The listing builds one solid part. Answer for the finished solid, in the listing's coordinates (mm). Face numbers are marked on the shaded views. A direction names the side the tool comes from. Give positions to 0.01 mm unless a question says otherwise; leave off trailing zeros. Order: outer loops, then holes, each group sorted by start corner. A loop starts at its lowest first (then second) coordinate and runs counter-clockwise, first axis right, second up. Notation, with made-up numbers: (-19, 64) - (-9, 64) arc R12 ccw to (-9, 80) - close; hole circle Ø11 at (13.25, -21). An arc over 180 degrees is marked (long way). Use CSV: the item, a comma, the result in double quotes.
```python
from build123d import *

# Parameters (mm, degrees)
FILLET1_R                     = 1
CHAMFER1_SIZE                 = 1.016
CHAMFER2_SIZE                 = 0.5
F_10_32_TAPPED_HOLE1_D        = 4.0386
F_10_32_TAPPED_HOLE1_DEPTH    = 13.6144
F_10_32_TAPPED_HOLE1_TIP      = 1.213317848
CUT_EXTRUDE1_START            = -6.79958
CUT_EXTRUDE1_DEPTH            = 122.301029095
SKETCH5_R                     = 4.318
BOSS_EXTRUDE1_DEPTH           = 2.2606
BOSS_EXTRUDE1_DRAFT           = 45
BOSS_EXTRUDE1_PROFILE_2_DEPTH = 2.2606
BOSS_EXTRUDE1_PROFILE_2_DRAFT = 45


with BuildPart() as part:
    # Sketch1 → Revolve1 (revolve)
    with BuildSketch(Plane(origin=(0, 0, 0), x_dir=(0, 0, -1), z_dir=(1, 0, 0)), mode=Mode.PRIVATE) as revolve1_sk:
        Polygon((-31.623, 0), (-31.623, 3.9751), (0, 3.9751), (0, 9.525), (3.9878, 9.525), (3.9878, 31.877), (12.2174, 31.877), (12.2174, 32.2072), (105.3592, 32.2072), (105.3592, 31.877), (113.5888, 31.877), (113.5888, 15.0368), (118.5888, 15.0368), (118.5888, 0), align=None)
    revolve(revolve1_sk.sketch.rotate(Axis((0, 0, 111.866494726), (0, 0, -1)), 90), axis=Axis((0, 0, 111.866494726), (0, 0, -1)))

    # Fillet1
    fillet1_edges = [part.edges().sort_by_distance(p)[0] for p in [
        (-31.877, 0, -113.5888),
        (-31.877, 0, -3.9878),
    ]]
    fillet(fillet1_edges, radius=FILLET1_R)

    # Chamfer1
    chamfer1_edges = [part.edges().sort_by_distance(p)[0] for p in [
        (-9.525, 0, 0),
        (-15.0368, 0, -118.5888),
    ]]
    chamfer(chamfer1_edges, length=CHAMFER1_SIZE)

    # Chamfer2
    chamfer2_edges = [part.edges().sort_by_distance(p)[0] for p in [
        (-3.9751, 0, 31.623),
    ]]
    chamfer(chamfer2_edges, length=CHAMFER2_SIZE)

    # #10-32 Tapped Hole1
    with Locations(Plane.XY):
        with Locations((0, 25.4), (0, -25.4)):
            Hole(F_10_32_TAPPED_HOLE1_D / 2, depth=F_10_32_TAPPED_HOLE1_DEPTH)
            with Locations((0, 0, -(F_10_32_TAPPED_HOLE1_DEPTH + F_10_32_TAPPED_HOLE1_TIP / 2))):  # 118° drill point
                Cone(0, F_10_32_TAPPED_HOLE1_D / 2, F_10_32_TAPPED_HOLE1_TIP, mode=Mode.SUBTRACT)

    # Sketch4 → Cut-Extrude1 (cut, through all)
    with BuildSketch(Plane(origin=(0, -3.9751, 0), x_dir=(-1, 0, 0), z_dir=(0, -1, 0)).offset(CUT_EXTRUDE1_START)):
        with BuildLine():
            Line((0.99949, -6.99389), (0.99949, -25.09393))
            ThreePointArc((0.99949, -25.09393), (0, -26.09342), (-0.99949, -25.09393))
            Line((-0.99949, -25.09393), (-0.99949, -6.99389))
            ThreePointArc((-0.99949, -6.99389), (0, -5.9944), (0.99949, -6.99389))
        make_face()
    extrude(amount=-CUT_EXTRUDE1_DEPTH, mode=Mode.SUBTRACT)


with BuildPart() as boss_extrude1_tool:
    # Sketch5 → Boss-Extrude1 (with draft: the straight prism first)
    with BuildSketch(Plane(origin=(0, 0, -113.5888), x_dir=(-1, 0, 0), z_dir=(0, 0, -1))):
        with Locations((11.185081873, 18.615102269)):
            Circle(SKETCH5_R)
    extrude(amount=BOSS_EXTRUDE1_DEPTH)
    # Boss-Extrude1: the draft: its side faces are tilted about the plane it starts from
    boss_extrude1_sides = [boss_extrude1_tool.faces().sort_by_distance(p)[0] for p in [
        (-6.867081873, 18.615102269, -114.7191),
    ]]
    draft(boss_extrude1_sides, Plane(origin=(0, 0, -113.5888), x_dir=(-1, 0, 0), z_dir=(0, 0, -1)), BOSS_EXTRUDE1_DRAFT)


with BuildPart() as part_1:
    add(part.part)

    # Boss-Extrude1: add boss_extrude1_tool
    add(boss_extrude1_tool.part)


with BuildPart() as boss_extrude1_profile_2_tool:
    # Sketch5 → Boss-Extrude1 profile 2 (with draft: the straight prism first)
    with BuildSketch(Plane(origin=(0, 0, -113.5888), x_dir=(-1, 0, 0), z_dir=(0, 0, -1))):
        with Locations((18.615102269, 11.185081873)):
            Circle(SKETCH5_R)
    extrude(amount=BOSS_EXTRUDE1_PROFILE_2_DEPTH)
    # Boss-Extrude1 profile 2: the draft: its side faces are tilted about the plane it starts from
    boss_extrude1_profile_2_sides = [boss_extrude1_profile_2_tool.faces().sort_by_distance(p)[0] for p in [
        (-14.297102269, 11.185081873, -114.7191),
    ]]
    draft(boss_extrude1_profile_2_sides, Plane(origin=(0, 0, -113.5888), x_dir=(-1, 0, 0), z_dir=(0, 0, -1)), BOSS_EXTRUDE1_PROFILE_2_DRAFT)


with BuildPart() as part_2:
    add(part_1.part)

    # Boss-Extrude1 profile 2: add boss_extrude1_profile_2_tool
    add(boss_extrude1_profile_2_tool.part)


solid = part_2.part
```
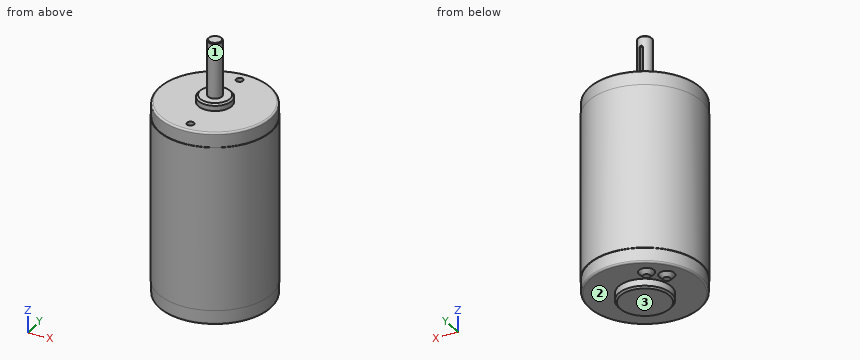
Item 1: Each of these flat-tipped pins is pushed along its axis until it touches: pin 1 (5 mm diameter, centred on y = 15, z = -79.5, fed in from +X); pin 2 (1.6 mm diameter, centred on x = 0, z = 15, fed in from +Y); pin 3 (4 mm diameter, centred on x = -22.5, y = -8, fed in from +Z). Where does it stop, or does it pass through?
Taken from the geometry:
pin 1,"x = 29.68"
pin 2,"y = 2.82"
pin 3,"z = -3.99"
Item 2: Which of the six approach directions +Z, -Z, +X, -X, +Y, -Y give full straight-line access (tool end or side, diameter ignored) to the marked faces 1, 2 and 3?
Taken from the geometry:
face 1,"+Z"
face 2,"-Z"
face 3,"-Z, +X, -X, +Y, -Y"
Item 3: Find the intervals of material crossed by line 1 along Y through (x, z) = (0, -8); line 2 along Z through (x, y) = (-27, -3.5); line 3 along X through (y, z) = (25.4, -6.25), in increasing order.
Taken from the geometry:
line 1,"-31.88 to -27.42, -23.38 to 23.38, 27.42 to 31.88"
line 2,"-113.59 to -3.99"
line 3,"-19.26 to -2.02, 2.02 to 19.26"
Item 4: The part is cut by section C-C (z = -100). Give the vertices of the cut face in (x, y), and give its area (3 significant figures).
Taken from the geometry:
outline,"circle Ø64.41 at (0, 0)"
area,"3,260 mm^2"
Item 5: The part is cut by section B-B (z = 15.5). Give the vertices of the cut face in (x, y).
Taken from the geometry:
outline,"(-1, 2.82) - (-1, 3.85) arc R3.98 ccw (long way) to (1, 3.85) - (1, 2.82) - close"
